Build history of the part. All positions in model axes, mm. Face numbers are marked on the shaded views. Round coordinates to 2 decimals unless told otherwise and drop trailing zeros. Write each loop counter-clockwise with the first axis right and the second up, starting at its lowest first coordinate (ties: lowest second). Pieces come first, ordered by that corner, then holes. Notation, with made-up numbers: (-31.75, 25.5) - (-6.75, 25.5) arc R22 cw to (-6.75, 49.5) - close; hole circle Ø10 at (67, 83.25). An arc over 180 degrees is marked (long way). One line per question, with ' | ' between items.
from build123d import *

# Parameters (mm, degrees)
F0_W     = 258.6008906364
F0_H     = 162.0002239943
F1_DEPTH = 9
F3_DEPTH = 330.2
F5_DEPTH = 190.5
F6_R     = 5
F7_START = 8
F7_DEPTH = 2


with BuildPart() as f1:
    # F0 (on Top) → F1 (new body)
    with BuildSketch(Plane.XY):
        Polygon((-141, -97.0001119971), (141, -97.0001119971), (147.5504453182, -97.0001119971), (147.5504453182, -92.0001119971), (147.5504453182, 97.0001119971), (141, 97.0001119971), (-141, 97.0001119971), (-147.5504453182, 97.0001119971), (-147.5504453182, -92.0001119971), (-147.5504453182, -97.0001119971), align=None)
        Polygon((145.3004453182, -95.0001119971), (138.75, -95.0001119971), (-138.75, -95.0001119971), (-145.3004453182, -95.0001119971), (-145.3004453182, -90.0001119971), (-145.3004453182, 95.0001119971), (-138.75, 95.0001119971), (138.75, 95.0001119971), (145.3004453182, 95.0001119971), (145.3004453182, -90.0001119971), align=None, mode=Mode.SUBTRACT)
        Polygon((-138.75, -95.0001119971), (138.75, -95.0001119971), (145.3004453182, -95.0001119971), (145.3004453182, -90.0001119971), (145.3004453182, 95.0001119971), (138.75, 95.0001119971), (-138.75, 95.0001119971), (-145.3004453182, 95.0001119971), (-145.3004453182, -90.0001119971), (-145.3004453182, -95.0001119971), align=None)
        Rectangle(F0_W, F0_H, mode=Mode.SUBTRACT)
        Rectangle(F0_W, F0_H)
    extrude(amount=F1_DEPTH)

    # F2 (on face) → F3 (cut)
    with BuildSketch(Plane.YZ.offset(147.5504453182)):
        Polygon((97.0001119971, 9), (95.0001119971, 0), (97.0001119971, 0), align=None)
        Polygon((-97.0001119971, 0), (-95.0001119971, 0), (-97.0001119971, 9), align=None)
    extrude(amount=-F3_DEPTH, mode=Mode.SUBTRACT)

    # F4 (on Front) → F5 (cut, symmetric)
    with BuildSketch(Plane.XZ):
        Polygon((-147.5504453182, 0), (-145.3004453182, 0), (-147.5504453182, 9), align=None)
        Polygon((147.5504453182, 9), (145.3004453182, 0), (147.5504453182, 0), align=None)
    extrude(amount=F5_DEPTH, both=True, mode=Mode.SUBTRACT)

    # F6
    f6_edges = [f1.edges().sort_by_distance(p)[0] for p in [
        (146.425445, -96.000112, 4.5),
        (-146.425445, -96.000112, 4.5),
        (146.425445, 96.000112, 4.5),
        (-146.425445, 96.000112, 4.5),
    ]]
    fillet(f6_edges, radius=F6_R)

    # F0 (on Top) → F7 (cut)
    with BuildSketch(Plane.XY.offset(F7_START)):
        Rectangle(F0_W, F0_H)
    extrude(amount=F7_DEPTH, mode=Mode.SUBTRACT)


solid = f1.part
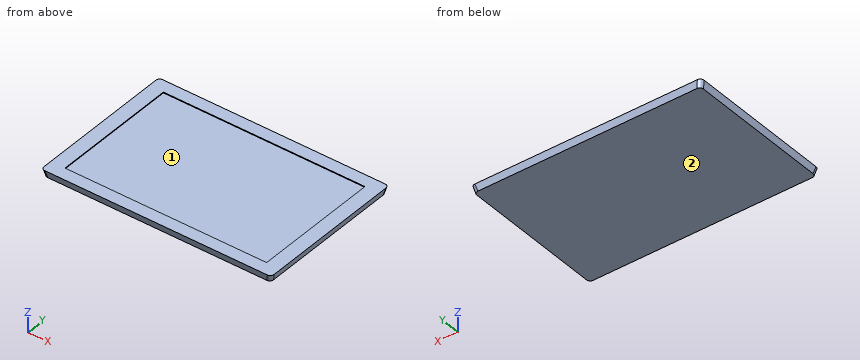
Q1. Drill centre lines: L1, parallel to Z at x = -52.5, y = 72.5; L2, parallel to Y at x = -29, z = 8.5; L3, parallel to X at y = 9, z = 4.5. Where is each one in solid material? Low to high. Write a range as from..to.
Found:
L1: 0..8 | L2: -96.89..-81, 81..96.89 | L3: -146.43..146.43
Q2. Drop flat-ended pins along their axis: pin 1 (3 mm diameter, centred on y = 76.5, z = 1, fed in from +X); pin 2 (1 mm diameter, centred on y = -76, z = 7.5, fed in from -X); pin 3 (0.8 mm diameter, centred on y = -14, z = 8.5, fed in from +X). Give the stop position or say it passes through.
Found:
pin 1: x = 145.93 | pin 2: x = -147.3 | pin 3: x = 147.53
Q3. Saw through at B-B, the plane x = 64.5. List the corners of the cut face in (y, z).
Found:
outline: (-97, 9) - (-95, 0) - (95, 0) - (97, 9) - (81, 9) - (81, 8) - (-81, 8) - (-81, 9) - close
Q4. Saw through at A-A, the plane y = 42. List the corners of the cut face in (x, z), then the cut area to 3 significant figures.
Found:
outline: (-147.55, 9) - (-145.3, 0) - (145.3, 0) - (147.55, 9) - (129.3, 9) - (129.3, 8) - (-129.3, 8) - (-129.3, 9) - close | area: 2,380 mm^2
Q5. Pull direction X, two halves, no side cores. Call the marked faces 1 and 2: +X half, -X half, draft (parallel to the pull), parting line (faces both ways), or undercut.
Found:
face 1: undercut | face 2: draft
